Work out the finished part from the listing and answer in its coordinate system (mm). A direction names the side the tool comes from. Coordinates: 2 decimals unless noted, no trailing zeros. Loops run counter-clockwise (first coordinate to the right, second up) from the corner with the lowest first, then second, coordinate; pieces in that order, holes last. Notation, with made-up numbers: (38.5, 73) -> (56.5, 73) arc R30 cw to (56.5, 102) -> close; hole circle Ø6 at (79, 87.25). An arc over 180 degrees is marked (long way). Use a Markdown table: item, result.
from build123d import *

# Parameters (mm, degrees)
CROQUIS1_W              = 40
CROQUIS1_H              = 50.135716494
SALIENTE_EXTRUIR1_DEPTH = 20
CROQUIS2_W              = 25
CROQUIS2_H              = 9.3
CORTAR_EXTRUIR1_DEPTH   = 41.703747176
CROQUIS3_W              = 25
CROQUIS3_H              = 9.3
CORTAR_EXTRUIR2_DEPTH   = 41.703747176
CORTAR_EXTRUIR3_DEPTH   = 41.703747176
CROQUIS5_W              = 12.7
CROQUIS5_H              = 20
TALADRO1_D              = 6.35
TALADRO1_DEPTH          = 15
TALADRO2_D              = 6.35
TALADRO2_DEPTH          = 15
CROQUIS11_W             = 20
CROQUIS11_H             = 12.953152015
CROQUIS11_H_2           = 13.688922843
SALIENTE_EXTRUIR2_DEPTH = 5
CROQUIS12_W             = 15
CROQUIS12_H             = 20
SALIENTE_EXTRUIR3_DEPTH = 5
CORTAR_EXTRUIR4_START   = -76
CROQUIS13_R             = 3.175
CORTAR_EXTRUIR4_DEPTH   = 76
CROQUIS14_W             = 15
CROQUIS14_H             = 20
SALIENTE_EXTRUIR4_DEPTH = 5
CROQUIS15_R             = 3.175
CORTAR_EXTRUIR5_DEPTH   = 72
CROQUIS16_W             = 30
CROQUIS16_H             = 20
SALIENTE_EXTRUIR5_DEPTH = 5
CROQUIS17_W             = 30
CROQUIS17_H             = 20
SALIENTE_EXTRUIR6_DEPTH = 5
CROQUIS20_W             = 20
CROQUIS20_H             = 17.953152015
CROQUIS20_H_2           = 18.688922843
SALIENTE_EXTRUIR7_DEPTH = 3
CROQUIS21_R             = 16.75
CORTAR_EXTRUIR8_DEPTH   = 43


with BuildPart() as part:
    # Croquis1 → Saliente-Extruir1 (new body)
    with BuildSketch(Plane(origin=(0, 0, 0), x_dir=(-1, 0, 0), z_dir=(0, 0, -1))):
        with Locations((5.067858247, 0)):
            Rectangle(CROQUIS1_W, CROQUIS1_H)
    extrude(amount=-SALIENTE_EXTRUIR1_DEPTH)

    # Croquis2 → Cortar-Extruir1 (cut, through all)
    with BuildSketch(Plane.XY.offset(20)):
        with Locations((2.432141753, -20.417858247)):
            Rectangle(CROQUIS2_W, CROQUIS2_H)
    extrude(amount=-CORTAR_EXTRUIR1_DEPTH, mode=Mode.SUBTRACT)

    # Croquis3 → Cortar-Extruir2 (cut, through all)
    with BuildSketch(Plane.XY.offset(20)):
        with Locations((2.432141753, 20.417858247)):
            Rectangle(CROQUIS3_W, CROQUIS3_H)
    extrude(amount=-CORTAR_EXTRUIR2_DEPTH, mode=Mode.SUBTRACT)

    # Croquis4 → Cortar-Extruir3 (cut, through all)
    with BuildSketch(Plane.XY.offset(20)):
        with BuildLine():
            Line((14.932141753, 2.814706232), (12.384160401, 2.814706232))
            ThreePointArc((12.384160401, 2.814706232), (12.694464867, 0.374915654), (12.528688183, -2.078935404))
            Line((12.528688183, -2.078935404), (14.932141753, -2.078935404))
            Line((14.932141753, -2.078935404), (14.932141753, 2.814706232))
        make_face()
    extrude(amount=-CORTAR_EXTRUIR3_DEPTH, mode=Mode.SUBTRACT)

    # Croquis5 → Cortar-Revolución1 (revolve, cut)
    with BuildSketch(Plane.XZ):
        with Locations((6.35, 10)):
            Rectangle(CROQUIS5_W, CROQUIS5_H)
    revolve(axis=Axis((0, 0, 20), (0, 0, -1)), mode=Mode.SUBTRACT)

    # Taladro1
    with Locations(Plane(origin=(0, -25.067858247, 0), x_dir=(-1, 0, 0), z_dir=(0, -1, 0))):
        with Locations((17.567858247, -9.999290914)):
            Hole(TALADRO1_D / 2, depth=TALADRO1_DEPTH)

    # Taladro2
    with Locations(Plane(origin=(0, 25.067858247, 0), x_dir=(1, 0, 0), z_dir=(0, 1, 0))):
        with Locations((-17.567858247, -10)):
            Hole(TALADRO2_D / 2, depth=TALADRO2_DEPTH)

    # Croquis11 → Saliente-Extruir2 (add)
    with BuildSketch(Plane(origin=(14.932141753, 0, 0), x_dir=(0, 0, -1), z_dir=(1, 0, 0))):
        with Locations((-10, 9.29128224)):
            Rectangle(CROQUIS11_W, CROQUIS11_H)
        with Locations((-10, -8.923396826)):
            Rectangle(CROQUIS11_W, CROQUIS11_H_2)
    extrude(amount=SALIENTE_EXTRUIR2_DEPTH)

    # Croquis12 → Saliente-Extruir3 (add)
    with BuildSketch(Plane(origin=(0, 25.067858247, 0), x_dir=(1, 0, 0), z_dir=(0, 1, 0))):
        with Locations((-17.567858247, -10)):
            Rectangle(CROQUIS12_W, CROQUIS12_H)
    extrude(amount=SALIENTE_EXTRUIR3_DEPTH)

    # Croquis13 → Cortar-Extruir4 (cut)
    with BuildSketch(Plane.XZ.offset(25.067858247).offset(CORTAR_EXTRUIR4_START)):
        with Locations(Location((-17.567858247, 9.999290914, 0), (0, 0, 270))):
            Circle(CROQUIS13_R)
    extrude(amount=CORTAR_EXTRUIR4_DEPTH, mode=Mode.SUBTRACT)

    # Croquis14 → Saliente-Extruir4 (add)
    with BuildSketch(Plane.XZ.offset(25.067858247)):
        with Locations((-17.567858247, 10)):
            Rectangle(CROQUIS14_W, CROQUIS14_H)
    extrude(amount=SALIENTE_EXTRUIR4_DEPTH)

    # Croquis15 → Cortar-Extruir5 (cut)
    with BuildSketch(Plane(origin=(0, 30.067858247, 0), x_dir=(1, 0, 0), z_dir=(0, 1, 0))):
        with Locations((-17.567858247, -9.999290914)):
            Circle(CROQUIS15_R)
    extrude(amount=-CORTAR_EXTRUIR5_DEPTH, mode=Mode.SUBTRACT)

    # Croquis16 → Saliente-Extruir5 (add)
    with BuildSketch(Plane(origin=(0, 15.767858247, 0), x_dir=(1, 0, 0), z_dir=(0, 1, 0))):
        with Locations((4.932141753, -10)):
            Rectangle(CROQUIS16_W, CROQUIS16_H)
    extrude(amount=SALIENTE_EXTRUIR5_DEPTH)

    # Croquis17 → Saliente-Extruir6 (add)
    with BuildSketch(Plane.XZ.offset(15.767858247)):
        with Locations((4.932141753, 10)):
            Rectangle(CROQUIS17_W, CROQUIS17_H)
    extrude(amount=SALIENTE_EXTRUIR6_DEPTH)

    # Croquis20 → Saliente-Extruir7 (add)
    with BuildSketch(Plane(origin=(19.932141753, 0, 0), x_dir=(0, 0, -1), z_dir=(1, 0, 0))):
        with Locations((-10, 11.79128224)):
            Rectangle(CROQUIS20_W, CROQUIS20_H)
        with Locations((-10, -11.423396826)):
            Rectangle(CROQUIS20_W, CROQUIS20_H_2)
    extrude(amount=SALIENTE_EXTRUIR7_DEPTH)

    # Croquis21 → Cortar-Extruir8 (cut)
    with BuildSketch(Plane.XY.offset(20)):
        with Locations((4.18967344, 0)):
            Circle(CROQUIS21_R)
    extrude(amount=-CORTAR_EXTRUIR8_DEPTH, mode=Mode.SUBTRACT)


solid = part.part
Q1. Section A-A on x = 13.5 is taken. Determine the outline of the cut face in (y, z).
Solved:
| item | result |
|---|---|
| outline | (-20.77, 0) -> (-13.92, 0) -> (-13.92, 20) -> (-20.77, 20) -> close; (13.92, 0) -> (20.77, 0) -> (20.77, 20) -> (13.92, 20) -> close |
Q2. For faces 4 (the flat face through (22, -2.079, 10)), 5 (the flat face through (6, 20.768, 10)), 6 (the flat face through (6, -20.768, 10)), determine the directions among +Z, -Z, +X, -X, +Y, -Y from which every point of the face is accessible in a straight line to the end or side of a thin tool.
Solved:
| item | result |
|---|---|
| face 4 | +Z, -Z, +X |
| face 5 | +Z, -Z, +X, +Y |
| face 6 | +Z, -Z, +X, -Y |
Q3. Determine the mould class of faces 1 (the flat face through (-14, 30.068, 10)), 2 (the cylindrical face through (4.702, -16.742, 10.14)), 3 (the flat face through (22.932, -11, 10)) for opening direction X: pulls with the +X half, pulls with the -X half, needs draft (parallel to the pull), parting line crosses it, or undercut.
Solved:
| item | result |
|---|---|
| face 1 | needs draft |
| face 2 | undercut |
| face 3 | pulls with the +X half |
Q4. Section D-D on z = 8 is taken. Determine the outline of the cut face in (x, y), and give its area (3 significant figures).
Solved:
| item | result |
|---|---|
| outline | (-25.07, -30.07) -> (-20.03, -30.07) -> (-20.03, 30.07) -> (-25.07, 30.07) -> close; (-15.1, -30.07) -> (-10.07, -30.07) -> (-10.07, -20.77) -> (22.93, -20.77) -> (22.93, -2.08) -> (20.81, -2.08) arc R16.75 cw to (-12.14, -3.73) arc R12.7 cw to (-12.14, 3.73) arc R16.75 cw to (20.7, 2.81) -> (22.93, 2.81) -> (22.93, 20.77) -> (-10.07, 20.77) -> (-10.07, 30.07) -> (-15.1, 30.07) -> close |
| area | 1,080 mm² |
Q5. Section C-C on y = 7.5 is taken. Determine the outline of the cut face in (x, z) (3 decimals), and give its area (3 significant figures).
Solved:
| item | result |
|---|---|
| outline | (-25.068, 0) -> (-10.787, 0) -> (-10.787, 20) -> (-25.068, 20) -> close; (19.167, 0) -> (22.932, 0) -> (22.932, 20) -> (19.167, 20) -> close; hole circle Ø6.35 at (-17.568, 9.999) |
| area | 329 mm² |
Q6. Section B-B on z = 17.5 is taken. Determine the outline of the cut face in (x, y), and give its area (3 significant figures).
Solved:
| item | result |
|---|---|
| outline | (-25.07, -30.07) -> (-10.07, -30.07) -> (-10.07, -20.77) -> (22.93, -20.77) -> (22.93, -2.08) -> (20.81, -2.08) arc R16.75 cw to (-12.14, -3.73) arc R12.7 cw to (-12.14, 3.73) arc R16.75 cw to (20.7, 2.81) -> (22.93, 2.81) -> (22.93, 20.77) -> (-10.07, 20.77) -> (-10.07, 30.07) -> (-25.07, 30.07) -> close |
| area | 1,380 mm² |
Q7. Given pin 1 Ø2 at (y, z) = (22.5, 16.5) entering from +X; pin 2 Ø0.7 at (x, z) = (22, 12.5) entering from -Y; pin 3 Ø0.6 at (x, z) = (21.5, 6.5) entering from +Y, each flat-ended and moving along its own axis, determine where each tip first touches the part or whether it passes through.
Solved:
| item | result |
|---|---|
| pin 1 | x = -10.07 |
| pin 2 | y = -20.77 |
| pin 3 | y = 20.77 |
Q8. Consider line 1 (X direction, y = 22, z = 19); line 2 (X direction, y = -5, z = 8.25); line 3 (Y direction, x = 18, z = 2). Determine where each line is inside the solid, lowest interval first. Write a range as [from, to].
Solved:
| item | result |
|---|---|
| line 1 | [-25.07, -10.07] |
| line 2 | [-25.07, -20.22], [-14.92, -11.8], [20.18, 22.93] |
| line 3 | [-20.77, -9.48], [9.48, 20.77] |
